Autodesk Inventor part; units mm, degrees
ref_plane "YZ Plane" through (0, 0, 0) normal (1, 0, 0) x (0, 1, 0)
ref_plane "XZ Plane" through (0, 0, 0) normal (0, 1, 0) x (-1, 0, 0)
ref_plane "XY Plane" through (0, 0, 0) normal (0, 0, 1) x (1, 0, 0)
sketch "草图1" plane through (0, 0, 0) normal (0, 1, 0) x (-1, 0, 0)
  line L0 (0, 0) -> (-67, 0)
  line L1 (-67, 0) -> (-67, -67)
  line L2 (-67, -67) -> (0, -67)
  line L3 (0, -67) -> (0, 0)
  line L4 (-2, -2) -> (-65, -2)
  line L5 (-65, -2) -> (-65, -65)
  line L6 (-65, -65) -> (-2, -65)
  line L7 (-2, -65) -> (-2, -2)
  dimension "d0" = 67
  dimension "d1" = 67
  dimension "d2" = 2
extrude "拉伸1" add sketch "草图1" along normal blind 30
sketch "草图2" plane through (0, 30, 0) normal (0, 1, 0) x (1, 0, 0)
  line L0 (67, 67) -> (0, 67)
  line L1 (0, 0) -> (67, 0)
  line L2 (67, 0) -> (67, 67)
  line L3 (67, 67) -> (0, 67)
  line L4 (0, 67) -> (0, 0)
  line L5 (-2, -2) -> (69, -2)
  line L6 (69, -2) -> (69, 69)
  line L7 (69, 69) -> (-2, 69)
  line L8 (-2, 69) -> (-2, -2)
  dimension "d5" = 2
extrude "拉伸2" add sketch "草图2" along normal blind 25 contours L2 L1 L4 L0 | L8 L7 L6 L5
fillet "圆角1" radius 3.5 4 edges at (67, 15, 0) (67, 15, -67) (0, 15, 0) (0, 15, -67)
fillet "圆角2" radius 5 8 edges at (-2, 42.5, 2) (-2, 42.5, -69) (-2, 55, -33.5) (33.5, 55, 2) (69, 42.5, 2) (69, 55, -33.5) (69, 42.5, -69) (33.5, 55, -69)
properties part number "顶盖"
The model under review builds one solid part; all positions refer to its coordinate system, in mm. A direction names the side the tool comes from. Round coordinates to 2 decimals unless told otherwise and drop trailing zeros. Loops run counter-clockwise (first coordinate to the right, second up) from the corner with the lowest first, then second, coordinate; pieces in that order, holes last. Notation, with made-up numbers: M 87,56.25 L 144,56.25 A18 cw 144,64.25 Z; hole C 57.25,40.5 d5. An arc over 180 degrees is marked long. Answer as CSV lines item,"result". Start each with the question number.
Item 1: Consider section C-C (x = 59). Write out the cut boundary in (y, z).
Item 2: Mouldability with a two-part tool opening along X and no side actions: class faces 6 (the face through (36, 0, -66)), 7 (the face through (67, 15, -33)), 8 (the face through (33, 30, -34)) as released by +X, released by -X, zero draft, split by the parting line, or undercut.
Item 3: Insertion check: P1, Ø5, axis at x = 30.5, z = -40.5, coming from the -Y side; P2, Ø1.5, axis at y = 10.5, z = -44.5, coming from the +X side; P3, Ø9, axis at x = 26, y = 9, coming from the -Z side. Each pin has a flat end and moves straight along its axis. Give the tip position at first contact, or say it passes through.
Item 4: For faces 1 (the face through (2, 15, -34)), 2 (the face through (0, 15, -34)), 3 (the face through (1.05, 15.21, -66)), 4 (the face through (1, 15.21, -1.05)), 5 (the face through (33, 15, 0)), list the 3-axis set-ups (+Z, -Z, +X, -X, +Y, -Y) from which the entire face can be reached by the end or side of a thin tool; tool diameter is ignored.
Item 5: Wall thickness on line 1 (X direction, y = 29, z = -53); line 2 (Z direction, x = 21, y = 13.5); line 3 (Y direction, x = 10, z = -47): over which ranges is each line inside the solid? List them lowest first. Write a range as [from, to].
Item 6: Consider section B-B (z = -59.5). Write out the cut boundary in (x, y), then the cut area to 3 significant figures.
Item 7: Consider section A-A (y = 20). Write out the cut boundary in (x, z).
Answer:
1,outline,"M 0,-67 L 30,-67 L 30,-69 L 50,-69 A5 ccw 55,-64 L 55,-3 A5 ccw 50,2 L 30,2 L 30,0 L 0,0 L 0,-2 L 30,-2 L 30,-65 L 0,-65 Z"
2,face 6,"zero draft"
2,face 7,"released by +X"
2,face 8,"undercut"
3,P1,"stops at y = 30"
3,P2,"stops at x = 67"
3,P3,"stops at z = -67"
4,face 1,"-Y"
4,face 2,"+Z, -Z, -X, -Y"
4,face 3,"-Z, -X, -Y"
4,face 4,"+Z, -X, -Y"
4,face 5,"+Z, +X, -X, -Y"
5,line 1,"x = [0, 2], [65, 67]"
5,line 2,"z = [-67, -65], [-2, 0]"
5,line 3,"y = [30, 55]"
6,outline,"M -2,30 L 0,30 L 0,0 L 2,0 L 2,30 L 65,30 L 65,0 L 67,0 L 67,30 L 69,30 L 69,50 A5 ccw 64,55 L 3,55 A5 ccw -2,50 Z"
6,area,"1,880 mm^2"
7,outline,"M 0,-63.5 A3.5 ccw 3.5,-67 L 63.5,-67 A3.5 ccw 67,-63.5 L 67,-3.5 A3.5 ccw 63.5,0 L 3.5,0 A3.5 ccw 0,-3.5 Z; hole M 2,-65 L 65,-65 L 65,-2 L 2,-2 Z"
